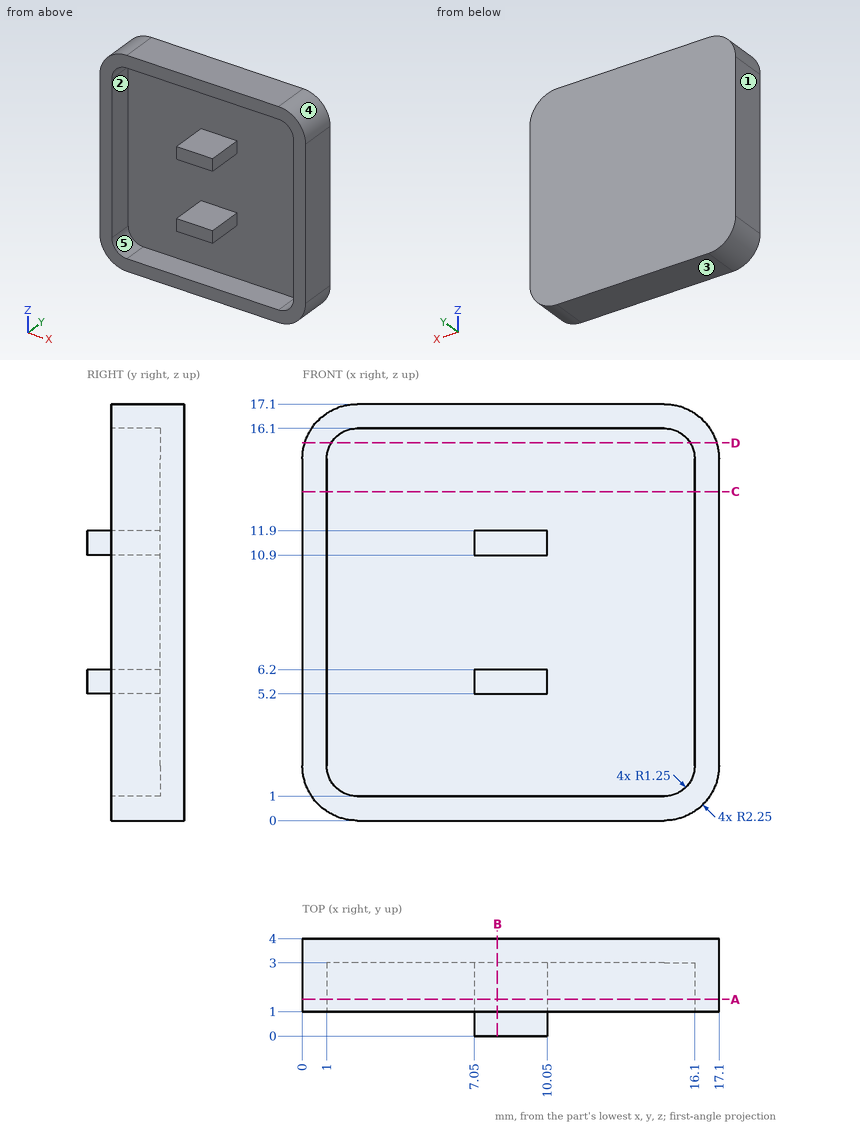
Design review of the part shown in the three views and the two pictorial views. Dimensions are in mm from the part's minimum x, y and z. A direction names the side the tool comes from. Round coordinates to 2 decimals unless told otherwise and drop trailing zeros. Order: outer loops, then holes, each group sorted by start corner. A loop starts at its lowest first (then second) coordinate and runs counter-clockwise, first axis right, second up.
Item 1: For pin 1 (7.5 mm diameter, centred on x = 10.5, z = 5, fed in from -Y), flat-tipped, find the tip position at first contact; note if it passes through.
Working result:
pin 1: stops at y = 0
Item 2: Add section B-B, the plane x = 8. State the section outline as (y, z) points, and give its area (3 significant figures).
Working result:
outline: (0, 5.2) - (3, 5.2) - (3, 1) - (1, 1) - (1, 0) - (4, 0) - (4, 17.1) - (1, 17.1) - (1, 16.1) - (3, 16.1) - (3, 11.9) - (0, 11.9) - (0, 10.9) - (3, 10.9) - (3, 6.2) - (0, 6.2) - close
area: 27.1 mm2
Item 3: To check wall thickness, follow probe 1 along Z at (x, y) = (8, 1.8); probe 2 along Z at (x, y) = (13, 2.1). State the ranges of each line that lie inside material, in increasing order.
Working result:
probe 1: z = 0 to 1, 5.2 to 6.2, 10.9 to 11.9, 16.1 to 17.1
probe 2: z = 0 to 1, 16.1 to 17.1
Item 4: Machinability: for the marked faces 1 and 2, which of the approach directions +Z, -Z, +X, -X, +Y, -Y give a long, thin tool a straight path to every point of the face, cutting with its end or side? Answer none if there is none.
Working result:
face 1: +Z, -Z, -X, +Y, -Y
face 2: -Y
Item 5: Add section D-D, the plane z = 15.5. State the section outline as (x, y) points, and give its area (3 significant figures).
Working result:
outline: (0.1, 1) - (1.18, 1) - (1.18, 3) - (15.92, 3) - (15.92, 1) - (17, 1) - (17, 4) - (0.1, 4) - close
area: 21.3 mm2
Item 6: Add section C-C, the plane z = 13.5. State the section outline as (x, y) points.
Working result:
outline: (0, 1) - (1, 1) - (1, 3) - (16.1, 3) - (16.1, 1) - (17.1, 1) - (17.1, 4) - (0, 4) - close
Item 7: Draft analysis for pull direction X (two halves, no side actions). For the marked faces 3, 4 and 5, state which applies: released by +X, released by -X, zero draft, split by the parting line, or undercut.
Working result:
face 3: zero draft
face 4: released by +X
face 5: undercut
Item 8: Add section A-A, the plane y = 1.5. State the section outline as (x, z) points, and give its area (3 significant figures).
Working result:
outline: (0, 2.25) arc R2.25 ccw to (2.25, 0) - (14.85, 0) arc R2.25 ccw to (17.1, 2.25) - (17.1, 14.85) arc R2.25 ccw to (14.85, 17.1) - (2.25, 17.1) arc R2.25 ccw to (0, 14.85) - close; (7.05, 5.2) - (10.05, 5.2) - (10.05, 6.2) - (7.05, 6.2) - close; (7.05, 10.9) - (10.05, 10.9) - (10.05, 11.9) - (7.05, 11.9) - close; hole (1, 2.25) arc R1.25 ccw to (2.25, 1) - (14.85, 1) arc R1.25 ccw to (16.1, 2.25) - (16.1, 14.85) arc R1.25 ccw to (14.85, 16.1) - (2.25, 16.1) arc R1.25 ccw to (1, 14.85) - close
area: 67.4 mm2
